Design review of the part built by this model. Coordinates are the model's own, in mm. Face numbers are marked on the shaded views. A direction names the side the tool comes from. Round coordinates to 2 decimals unless told otherwise and drop trailing zeros. Loops run counter-clockwise (first coordinate to the right, second up) from the corner with the lowest first, then second, coordinate; pieces in that order, holes last. Notation, with made-up numbers: (-7.75, -6) - (18.25, -6) arc R5 ccw to (18.25, 1) - close; hole circle Ø5 at (0, 25). An arc over 180 degrees is marked (long way). Return JSON: item names as keys, results as strings. Group by question number.
(1) Clearance check with flat-ended pins moving along their axes: pin 1 (6 mm diameter, centred on x = 30.5, y = 9.5, fed in from +Z); pin 2 (1.3 mm diameter, centred on y = 10, z = -10.5, fed in from +X); pin 3 (3 mm diameter, centred on x = 18.5, y = 8, fed in from +Z); pin 4 (13 mm diameter, centred on x = 11, z = -12, fed in from +Y). State where each tip first meets the part, or that it passes through.
(2) We need section A-A, the plane y = 9.75. Write out the cut boundary in (x, z).
(3) The part is to be moulded in two halves that separate along X. For the marked faces 1, 2 and 3, say which applies: pulls with the +X half, pulls with the -X half, needs draft (parallel to the pull), parting line crosses it, or undercut.
(4) Wall thickness on L1, parallel to Z at x = 23.5, y = 8.5; L2, parallel to Z at x = 35, y = 6; L3, parallel to X at y = 6, z = -16.5: over which ranges is each line inside the solid? List them lowest first. Write a range as [from, to].
(5) We need section D-D, the plane z = -16. Write out the cut boundary in (x, y).
(6) We need section C-C, the plane x = 29. Write out the cut boundary in (y, z), and give its area (3 significant figures).
(7) For the marked faces 4 and 5, list the 3-axis set-ups (+Z, -Z, +X, -X, +Y, -Y) from which the entire face can be reached by the end or side of a thin tool; tool diameter is ignored.
(8) We need section B-B, the plane z = -2. Write out the cut boundary in (x, y).
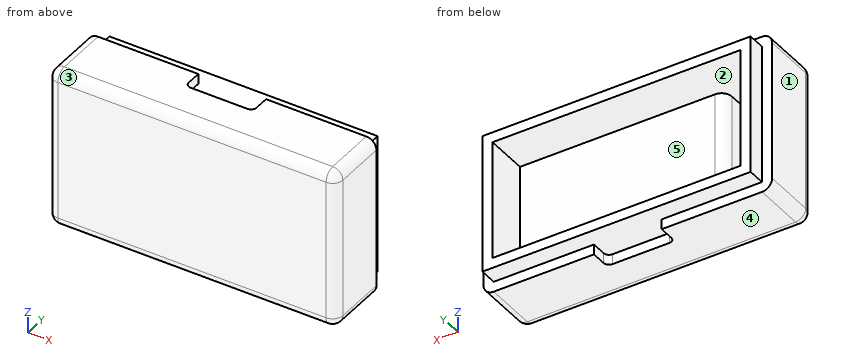
from build123d import *

# Parameters (mm, degrees)
SKETCH2_W           = 42.6
SKETCH2_H           = 23.6
BOSS_EXTRUDE1_DEPTH = 11.8
SKETCH4_W           = 30.3
SKETCH4_H           = 17.6
CUT_EXTRUDE2_DEPTH  = 6.3
SKETCH5_W           = 6.3
SKETCH5_H           = 17.6
CUT_EXTRUDE3_DEPTH  = 10.3
SKETCH6_W           = 42.6
SKETCH6_H           = 23.6
SKETCH6_W_2         = 39.6
SKETCH6_H_2         = 20.6
CUT_EXTRUDE4_DEPTH  = 2.6
FILLET1_R           = 1.5
FILLET2_R           = 1.5
CUT_EXTRUDE5_DEPTH  = 1.5
CUT_EXTRUDE6_START  = -1.5
CUT_EXTRUDE6_DEPTH  = 1.5


with BuildPart() as part:
    # Sketch2 → Boss-Extrude1 (new body)
    with BuildSketch(Plane(origin=(0, 0, 0), x_dir=(1, 0, 0), z_dir=(0, 1, 0))):
        with Locations((21.3, 11.8)):
            Rectangle(SKETCH2_W, SKETCH2_H)
    extrude(amount=BOSS_EXTRUDE1_DEPTH)

    # Sketch4 → Cut-Extrude2 (cut)
    with BuildSketch(Plane(origin=(0, 11.8, 0), x_dir=(1, 0, 0), z_dir=(0, 1, 0))):
        with Locations((24.45, 11.8)):
            Rectangle(SKETCH4_W, SKETCH4_H)
    extrude(amount=-CUT_EXTRUDE2_DEPTH, mode=Mode.SUBTRACT)

    # Sketch5 → Cut-Extrude3 (cut)
    with BuildSketch(Plane(origin=(0, 11.8, 0), x_dir=(1, 0, 0), z_dir=(0, 1, 0))):
        with Locations((6.15, 11.8)):
            Rectangle(SKETCH5_W, SKETCH5_H)
    extrude(amount=-CUT_EXTRUDE3_DEPTH, mode=Mode.SUBTRACT)

    # Sketch6 → Cut-Extrude4 (cut)
    with BuildSketch(Plane(origin=(0, 11.8, 0), x_dir=(1, 0, 0), z_dir=(0, 1, 0))):
        with Locations((21.3, 11.8)):
            Rectangle(SKETCH6_W, SKETCH6_H)
        with Locations((21.3, 11.8)):
            Rectangle(SKETCH6_W_2, SKETCH6_H_2, mode=Mode.SUBTRACT)
    extrude(amount=-CUT_EXTRUDE4_DEPTH, mode=Mode.SUBTRACT)

    # Fillet1
    fillet1_edges = [part.edges().sort_by_distance(p)[0] for p in [
        (0, 4.6, -23.6),
        (42.6, 4.6, -23.6),
        (42.6, 4.6, 0),
        (0, 4.6, 0),
        (21.3, 0, -23.6),
        (42.6, 0, -11.8),
        (21.3, 0, 0),
        (0, 0, -11.8),
    ]]
    fillet(fillet1_edges, radius=FILLET1_R)

    # Fillet2
    fillet2_edges = [part.edges().sort_by_distance(p)[0] for p in [
        (9.3, 5.5, -11.8),
    ]]
    fillet(fillet2_edges, radius=FILLET2_R)

    # Sketch8 → Cut-Extrude5 (cut)
    with BuildSketch(Plane.XY):
        with BuildLine():
            Line((16.3, 9.2), (26.3, 9.2))
            Line((26.3, 9.2), (26.3, 7))
            ThreePointArc((26.3, 7), (26.065685425, 6.434314575), (25.5, 6.2))
            Line((25.5, 6.2), (17.1, 6.2))
            ThreePointArc((17.1, 6.2), (16.534314575, 6.434314575), (16.3, 7))
            Line((16.3, 7), (16.3, 9.2))
        make_face()
    extrude(amount=-CUT_EXTRUDE5_DEPTH, mode=Mode.SUBTRACT)

    # Sketch9 → Cut-Extrude6 (cut)
    with BuildSketch(Plane(origin=(0, 0, -23.6), x_dir=(-1, 0, 0), z_dir=(0, 0, -1)).offset(CUT_EXTRUDE6_START)):
        with BuildLine():
            Line((-16.3, 9.2), (-26.3, 9.2))
            Line((-26.3, 9.2), (-26.3, 7))
            ThreePointArc((-26.3, 7), (-26.065685425, 6.434314575), (-25.5, 6.2))
            Line((-25.5, 6.2), (-17.1, 6.2))
            ThreePointArc((-17.1, 6.2), (-16.534314575, 6.434314575), (-16.3, 7))
            Line((-16.3, 7), (-16.3, 9.2))
        make_face()
    extrude(amount=CUT_EXTRUDE6_DEPTH, mode=Mode.SUBTRACT)


solid = part.part
Solutions:
{
 "1": {"pin 1": "z = 0", "pin 2": "x = 41.1", "pin 3": "z = -1.5", "pin 4": "y = 5.5"},
 "2": {"outline": "(1.5, -22.1) - (41.1, -22.1) - (41.1, -1.5) - (1.5, -1.5) - close; hole (3, -20.6) - (39.6, -20.6) - (39.6, -3) - (3, -3) - close"},
 "3": {"face 1": "pulls with the -X half", "face 2": "undercut", "face 3": "needs draft"},
 "4": {"L1": "[-22.1, -20.6], [-3, -1.5]", "L2": "[-23.6, -20.6], [-3, 0]", "L3": "[0, 3], [39.6, 42.6]"},
 "5": {"outline": "(0, 1.5) arc R1.5 ccw to (1.5, 0) - (41.1, 0) arc R1.5 ccw to (42.6, 1.5) - (42.6, 9.2) - (41.1, 9.2) - (41.1, 11.8) - (39.6, 11.8) - (39.6, 5.5) - (10.8, 5.5) arc R1.5 ccw to (9.3, 4) - (9.3, 1.5) - (3, 1.5) - (3, 11.8) - (1.5, 11.8) - (1.5, 9.2) - (0, 9.2) - close"},
 "6": {"outline": "(0, -22.1) arc R1.5 ccw to (1.5, -23.6) - (9.2, -23.6) - (9.2, -22.1) - (11.8, -22.1) - (11.8, -20.6) - (5.5, -20.6) - (5.5, -3) - (11.8, -3) - (11.8, -1.5) - (9.2, -1.5) - (9.2, 0) - (1.5, 0) arc R1.5 ccw to (0, -1.5) - close", "area": "159 mm^2"},
 "7": {"face 4": "-Z, +X, -X, +Y, -Y", "face 5": "+Y"},
 "8": {"outline": "(0, 1.5) arc R1.5 ccw to (1.5, 0) - (41.1, 0) arc R1.5 ccw to (42.6, 1.5) - (42.6, 9.2) - (41.1, 9.2) - (41.1, 11.8) - (1.5, 11.8) - (1.5, 9.2) - (0, 9.2) - close"}
}
